```python
from build123d import *

# Parameters (mm, degrees)
ESBO_O1_R                     = 75
RESSALTO_EXTRUS_O1_DEPTH      = 1500
RESSALTO_EXTRUS_O2_DEPTH      = 200
RESSALTO_EXTRUS_O2_DEPTH_BACK = 200
ESBO_O2_R                     = 75
ESBO_O3_R                     = 400
RESSALTO_EXTRUS_O3_DEPTH      = 100
FILETE1_R                     = 90
FILETE1_OF_ESPELHAR1_R        = 90


with BuildPart() as part:
    # Esbo_o1 → Ressalto-extrus_o1 (new body)
    with BuildSketch(Plane(origin=(0, 0, 0), x_dir=(1, 0, 0), z_dir=(0, 1, 0))):
        with Locations(Location((0, 0, 0), (0, 0, 270))):
            Circle(ESBO_O1_R)
    extrude(amount=RESSALTO_EXTRUS_O1_DEPTH)

    # Esbo_o2 → Ressalto-extrus_o2 (add, two sides: drawn at the far end of the back side and taken through both)
    with BuildSketch(Plane.XY.offset(-RESSALTO_EXTRUS_O2_DEPTH_BACK)):
        Circle(ESBO_O2_R)
    extrude(amount=RESSALTO_EXTRUS_O2_DEPTH + RESSALTO_EXTRUS_O2_DEPTH_BACK)

    # Esbo_o3 → Ressalto-extrus_o3 (add, symmetric)
    with BuildSketch(Plane.XY.offset(200)):
        Circle(ESBO_O3_R)
    ressalto_extrus_o3 = extrude(amount=RESSALTO_EXTRUS_O3_DEPTH, both=True)

    # Filete1
    filete1_edges = [part.edges().sort_by_distance(p)[0] for p in [
        (-400, 0, 100),
        (-400, 0, 300),
    ]]
    fillet(filete1_edges, radius=FILETE1_R)

    # Espelhar1: Ressalto-extrus_o3 across plane
    add(ressalto_extrus_o3.mirror(Plane.XY))

    # Filete1 of Espelhar1
    filete1_of_espelhar1_edges = [part.edges().sort_by_distance(p)[0] for p in [
        (-400, 0, -100),
        (-400, 0, -300),
    ]]
    fillet(filete1_of_espelhar1_edges, radius=FILETE1_OF_ESPELHAR1_R)


solid = part.part
```
Here's how the part is built. I have some questions about the finished solid (model axes, mm). A direction names the side the tool comes from. Give positions to 0.01 mm unless a question says otherwise; leave off trailing zeros. Write each loop counter-clockwise with the first axis right and the second up, starting at its lowest first coordinate (ties: lowest second). Pieces come first, ordered by that corner, then holes. Notation, with made-up numbers: M 79,-16 L 134,-16 A35 cw 134,20 Z; hole C -9.75,49.25 d6. An arc over 180 degrees is marked long. Put each result on its own line as item: value. Start each with the question number.
Item 1: If we section it at A-A, the plane x = 0: Write out the boundary of the cut face in (y, z).
Item 2: Will these pins go through, and if not, where does the flat tip stop? pin 1 (12 mm diameter, centred on x = -84, y = 762.5, fed in from -Z); pin 2 (2 mm diameter, centred on y = 23.5, z = 34, fed in from -X); pin 3 (12 mm diameter, centred on y = 41, z = -72.5, fed in from -X); pin 4 (1 mm diameter, centred on x = 72, z = 186, fed in from +Y).
Item 3: If we section it at D-D, the plane z = 154: Write out the boundary of the cut face in (x, y), then the cut area to 3 significant figures.
Item 4: If we section it at C-C, the plane z = 0: Write out the boundary of the cut face in (x, y).
Item 5: I need wall thicknesses on L1, parallel to Z at x = -97, y = -138; L2, parallel to Y at x = 310.5, z = -263.5; L3, parallel to Z at x = 26, y = 615.5. Which ranges of each line are inside material? Lowest first, please. Write a range as from..to.
Item 6: If we section it at B-B, the plane y = 567.5: Write out the boundary of the cut face in (x, z), then the cut area to 3 significant figures.
Item 7: On a 3-axis mill with a long thin cutter (end or side, diameter ignored), from which of +Z, -Z, +X, -X, +Y, -Y can I reach the whole of each face in a straight line? I mean faces 1 (the flat face through (-4, 4, 300)), 2 (the cylindrical face through (-16.259, -73.217, -1.4)), 3 (the cylindrical face through (22.528, 739.5, 71.537)). Say none if no direction works.
Values:
1. outline: M -400,-210 A90 ccw -310,-300 L 310,-300 A90 ccw 400,-210 L 400,-190 A90 ccw 310,-100 L 75,-100 L 75,-75 L 1500,-75 L 1500,75 L 75,75 L 75,100 L 310,100 A90 ccw 400,190 L 400,210 A90 ccw 310,300 L -310,300 A90 ccw -400,210 L -400,190 A90 ccw -310,100 L -75,100 L -75,-100 L -310,-100 A90 ccw -400,-190 Z
2. pin 1: through
2. pin 2: x = -71.55
2. pin 3: x = -66.33
2. pin 4: y = 393.47
3. outline: C 0,0 d784.97
3. area: 484,000 mm²
4. outline: M -75,0 A75 ccw 75,0 L 75,1500 L -75,1500 Z
5. L1: -300..-100, 100..300
5. L2: -223.16..223.16
5. L3: -70.35..70.35
6. outline: C 0,0 d150
6. area: 17,700 mm²
7. face 1: +Z, +X, -X, +Y, -Y
7. face 2: none
7. face 3: +Y
